```python
from build123d import *

# Parameters (mm, degrees)
SKETCH_1_W          = 120
SKETCH_1_H          = 70
EXTRUDE_1_DEPTH     = 5
SKETCH_2_W          = 120
SKETCH_2_H          = 70
EXTRUDE_2_DEPTH     = 5
SKETCH_3_W          = 8
SKETCH_3_H          = 72
SKETCH_3_W_2        = 72
SKETCH_3_H_2        = 8
EXTRUDE_3_DEPTH     = 50
SKETCH_4_W          = 300
SKETCH_4_H          = 300
EXTRUDE_4_DEPTH     = 5
EXTRUDE_5_DEPTH     = 5
SKETCH_6_W          = 4
SKETCH_6_H          = 3
CUT_EXTRUDE_1_DEPTH = 3
SKETCH_7_R          = 0.4
CUT_EXTRUDE_2_DEPTH = 3
SKETCH_8_W          = 3
SKETCH_8_H          = 4
CUT_EXTRUDE_3_DEPTH = 3
SKETCH_9_R          = 0.4
CUT_EXTRUDE_4_DEPTH = 3


with BuildPart() as part:
    # 草图1 → 凸台-拉伸1 (new body)
    with BuildSketch(Plane(origin=(0, 0, 0), x_dir=(1, 0, 0), z_dir=(0, 1, 0))):
        Polygon((-150, 150), (150, 150), (150, -30), (150, -150), (0, -150), (-150, -150), align=None)
        Polygon((-15.857864376, 30), (120, 30), (120, -30), (44.142135624, -30), align=None, mode=Mode.SUBTRACT)
        Polygon((-105.857864376, 120), (120, 120), (120, 50), (-35.857864376, 50), align=None, mode=Mode.SUBTRACT)
        Polygon((-120, 105.857864376), (-120, 50), (-64.142135624, 50), align=None, mode=Mode.SUBTRACT)
        with Locations((-60, -85)):
            Rectangle(SKETCH_1_W, SKETCH_1_H, mode=Mode.SUBTRACT)
        Polygon((-120, 30), (-44.142135624, 30), (15.857864376, -30), (-120, -30), align=None, mode=Mode.SUBTRACT)
    extrude(amount=EXTRUDE_1_DEPTH)

    # 草图2 → 凸台-拉伸2 (add)
    with BuildSketch(Plane.XZ):
        with BuildLine():
            Line((150, 45), (150, 150))
            Line((150, 150), (-150, 150))
            Line((-150, 150), (-150, -150))
            Line((-150, -150), (150, -150))
            Line((150, -150), (150, -45))
            Line((150, -45), (-110, -45))
            ThreePointArc((-110, -45), (-111.913417162, -44.619397663), (-113.535533906, -43.535533906))
            ThreePointArc((-113.535533906, -43.535533906), (-115, -42.928932188), (-116.464466094, -43.535533906))
            ThreePointArc((-116.464466094, -43.535533906), (-125, -40), (-116.464466094, -36.464466094))
            ThreePointArc((-116.464466094, -36.464466094), (-115, -37.071067812), (-113.535533906, -36.464466094))
            ThreePointArc((-113.535533906, -36.464466094), (-111.913417162, -35.380602337), (-110, -35))
            Line((-110, -35), (150, -35))
            Line((150, -35), (150, 35))
            Line((150, 35), (-110, 35))
            ThreePointArc((-110, 35), (-111.913417162, 35.380602337), (-113.535533906, 36.464466094))
            ThreePointArc((-113.535533906, 36.464466094), (-115, 37.071067812), (-116.464466094, 36.464466094))
            ThreePointArc((-116.464466094, 36.464466094), (-125, 40), (-116.464466094, 43.535533906))
            ThreePointArc((-116.464466094, 43.535533906), (-115, 42.928932188), (-113.535533906, 43.535533906))
            ThreePointArc((-113.535533906, 43.535533906), (-111.913417162, 44.619397663), (-110, 45))
            Line((-110, 45), (150, 45))
        make_face()
        with Locations((-60, 85)):
            Rectangle(SKETCH_2_W, SKETCH_2_H, mode=Mode.SUBTRACT)
        Polygon((-120, 30), (-120, -30), (-44.142135624, -30), (15.857864376, 30), align=None, mode=Mode.SUBTRACT)
        Polygon((44.142135624, 30), (-15.857864376, -30), (120, -30), (120, 30), align=None, mode=Mode.SUBTRACT)
        Polygon((-120, -50), (-120, -105.857864376), (-64.142135624, -50), align=None, mode=Mode.SUBTRACT)
        Polygon((-35.857864376, -50), (-105.857864376, -120), (120, -120), (120, -50), align=None, mode=Mode.SUBTRACT)
    extrude(amount=EXTRUDE_2_DEPTH)

    # 草图3 → 凸台-拉伸3 (add)
    with BuildSketch(Plane(origin=(0, 5, 0), x_dir=(1, 0, 0), z_dir=(0, 1, 0))):
        with Locations((146, -106)):
            Rectangle(SKETCH_3_W, SKETCH_3_H)
        with Locations((-106, -146)):
            Rectangle(SKETCH_3_W_2, SKETCH_3_H_2)
        with Locations((-146, 106)):
            Rectangle(SKETCH_3_W, SKETCH_3_H)
        with Locations((106, 146)):
            Rectangle(SKETCH_3_W_2, SKETCH_3_H_2)
    extrude(amount=EXTRUDE_3_DEPTH)

    # 草图4 → 凸台-拉伸4 (add)
    with BuildSketch(Plane(origin=(0, 55, 0), x_dir=(1, 0, 0), z_dir=(0, 1, 0))):
        Rectangle(SKETCH_4_W, SKETCH_4_H)
        Polygon((30, 120), (-30, 120), (-30, -15.857864376), (30, 44.142135624), align=None, mode=Mode.SUBTRACT)
        Polygon((105.857864376, 120), (50, 120), (50, 64.142135624), align=None, mode=Mode.SUBTRACT)
        Polygon((120, 105.857864376), (120, -120), (50, -120), (50, 35.857864376), align=None, mode=Mode.SUBTRACT)
        Polygon((-120, 120), (-120, -105.857864376), (-50, -35.857864376), (-50, 120), align=None, mode=Mode.SUBTRACT)
        Polygon((-50, -120), (-105.857864376, -120), (-50, -64.142135624), align=None, mode=Mode.SUBTRACT)
        Polygon((30, -120), (-30, -120), (-30, -44.142135624), (30, 15.857864376), align=None, mode=Mode.SUBTRACT)
    extrude(amount=EXTRUDE_4_DEPTH)

    # 草图5 → 凸台-拉伸5 (add)
    with BuildSketch(Plane(origin=(0, 60, 0), x_dir=(1, 0, 0), z_dir=(0, 1, 0))):
        with BuildLine():
            Line((35, 110), (35, -150))
            Line((35, -150), (45, -150))
            Line((45, -150), (45, 110))
            ThreePointArc((45, 110), (44.619397663, 111.913417162), (43.535533906, 113.535533906))
            ThreePointArc((43.535533906, 113.535533906), (42.928932188, 115), (43.535533906, 116.464466094))
            ThreePointArc((43.535533906, 116.464466094), (40, 125), (36.464466094, 116.464466094))
            ThreePointArc((36.464466094, 116.464466094), (37.071067812, 115), (36.464466094, 113.535533906))
            ThreePointArc((36.464466094, 113.535533906), (35.380602337, 111.913417162), (35, 110))
        make_face()
        with BuildLine():
            Line((-45, -150), (-35, -150))
            Line((-35, -150), (-35, 110))
            ThreePointArc((-35, 110), (-35.380602337, 111.913417162), (-36.464466094, 113.535533906))
            ThreePointArc((-36.464466094, 113.535533906), (-37.071067812, 115), (-36.464466094, 116.464466094))
            ThreePointArc((-36.464466094, 116.464466094), (-40, 125), (-43.535533906, 116.464466094))
            ThreePointArc((-43.535533906, 116.464466094), (-42.928932188, 115), (-43.535533906, 113.535533906))
            ThreePointArc((-43.535533906, 113.535533906), (-44.619397663, 111.913417162), (-45, 110))
            Line((-45, 110), (-45, -150))
        make_face()
    extrude(amount=EXTRUDE_5_DEPTH)

    # 草图6 → 切除-拉伸1 (cut)
    with BuildSketch(Plane.XZ):
        with Locations((138, 42.5)):
            Rectangle(SKETCH_6_W, SKETCH_6_H)
        with Locations((138, 37.5)):
            Rectangle(SKETCH_6_W, SKETCH_6_H)
    extrude(amount=-CUT_EXTRUDE_1_DEPTH, mode=Mode.SUBTRACT)

    # 草图7 → 切除-拉伸2 (cut)
    with BuildSketch(Plane.XZ.offset(-3)):
        with Locations(Location((138, 43.5, 0), (0, 0, 270))):
            Circle(SKETCH_7_R)
        with Locations(Location((138, 41.5, 0), (0, 0, 90))):
            Circle(SKETCH_7_R)
        with Locations(Location((138, 36.5, 0), (0, 0, 90))):
            Circle(SKETCH_7_R)
        with Locations(Location((138, 38.5, 0), (0, 0, 270))):
            Circle(SKETCH_7_R)
    extrude(amount=-CUT_EXTRUDE_2_DEPTH, mode=Mode.SUBTRACT)

    # 草图8 → 切除-拉伸3 (cut)
    with BuildSketch(Plane(origin=(0, 65, 0), x_dir=(1, 0, 0), z_dir=(0, 1, 0))):
        with Locations((37.5, -138)):
            Rectangle(SKETCH_8_W, SKETCH_8_H)
        with Locations((42.5, -138)):
            Rectangle(SKETCH_8_W, SKETCH_8_H)
    extrude(amount=-CUT_EXTRUDE_3_DEPTH, mode=Mode.SUBTRACT)

    # 草图9 → 切除-拉伸4 (cut)
    with BuildSketch(Plane(origin=(0, 62, 0), x_dir=(1, 0, 0), z_dir=(0, 1, 0))):
        with Locations(Location((43.5, -138, 0), (0, 0, 270))):
            Circle(SKETCH_9_R)
        with Locations(Location((41.5, -138, 0), (0, 0, 270))):
            Circle(SKETCH_9_R)
        with Locations(Location((36.5, -138, 0), (0, 0, 90))):
            Circle(SKETCH_9_R)
        with Locations(Location((38.5, -138, 0), (0, 0, 90))):
            Circle(SKETCH_9_R)
    extrude(amount=-CUT_EXTRUDE_4_DEPTH, mode=Mode.SUBTRACT)


solid = part.part
```
Source: CAD feature listing. Evaluate the final solid. Frame: model axes, mm. A direction names the side the tool comes from. Give positions to 0.01 mm unless a question says otherwise; leave off trailing zeros. Loops run counter-clockwise (first coordinate to the right, second up) from the corner with the lowest first, then second, coordinate; pieces in that order, holes last. Notation, with made-up numbers: (-28.75, -7) -> (-2.75, -7) arc R29 cw to (-2.75, 27) -> close; hole circle Ø6 at (27, 67.5). An arc over 180 degrees is marked (long way). Use a Markdown table: item, result. Add a question column.
(1) Section query D-D (x = 131.5). Output: boundary loops of the cut face in (y, z).
(2) Section query B-B (x = 81). Count the separate pieces of the cut face and the enclosed holes in it, then the cut area to 3 significant figures.
(3) Ray query, line 1 (Z direction, x = 138, y = 4); line 2 (X direction, y = 60.45, z = 138). Return the intervals inside material, ascending.
(4) Access query for faces 1 (the face through (-2, 55, -2)), 2 (the face through (-142, 30, 146)), 3 (the face through (-120, 0, 0)). Directions: +Z, -Z, +X, -X, +Y, -Y. A direction counts if a zero-diameter tool reaches every point of the face in a straight line with its end or side. Return the directions, or none.
(5) Pull-direction query (X, two-part tool) for faces 4 (the face through (142, 30, -146)), 5 (the face through (-61, 0, 50)), 6 (the face through (-146, 30, -142)); classes: +X half, -X half, draft (parallel to the pull), parting line (faces both ways), or undercut.
(6) Section query A-A (y = 32.5). Output: boundary loops of the cut face in (x, z), then the cut area to 3 significant figures.
(7) First-contact query: pin 1 Ø9 at (y, z) = (21, -146) entering from -X; pin 2 Ø12 at (y, z) = (20, -91) entering from +X; pin 3 Ø0.9 at (x, z) = (138.5, 42) entering from -Y; pin 4 Ø3 at (x, y) = (-88, 23) entering from -Z. Flat tips, straight axial feed; report the tip coordinate or a pass-through.
Checked values:
| question | item | result |
|---|---|---|
| 1 | outline | (-5, -150) -> (60, -150) -> (60, 150) -> (55, 150) -> (55, -142) -> (5, -142) -> (5, 150) -> (-5, 150) -> (-5, 45) -> (0, 45) -> (0, 35) -> (-5, 35) -> (-5, -35) -> (0, -35) -> (0, -45) -> (-5, -45) -> close |
| 2 | separate pieces | 5 |
| 2 | enclosed holes | 0 |
| 2 | area | 2,440 mm^2 |
| 3 | line 1 | -150 to 36.1, 36.9 to 38.1, 38.9 to 41.1, 41.9 to 43.1, 43.9 to 150 |
| 3 | line 2 | -45 to -35, 35 to 36.1, 36.9 to 38.1, 38.9 to 41.1, 41.9 to 43.1, 43.9 to 45 |
| 4 | face 1 | none |
| 4 | face 2 | +Z, -X |
| 4 | face 3 | +Y, -Y |
| 5 | face 4 | +X half |
| 5 | face 5 | undercut |
| 5 | face 6 | draft |
| 6 | outline | (-150, -142) -> (-142, -142) -> (-142, -70) -> (-150, -70) -> close; (-142, 142) -> (-70, 142) -> (-70, 150) -> (-142, 150) -> close; (70, -150) -> (142, -150) -> (142, -142) -> (70, -142) -> close; (142, 70) -> (150, 70) -> (150, 142) -> (142, 142) -> close |
| 6 | area | 2,300 mm^2 |
| 7 | pin 1 | x = -150 |
| 7 | pin 2 | x = -142 |
| 7 | pin 3 | y = 3 |
| 7 | pin 4 | z = 142 |
